from build123d import *

# Parameters (mm, degrees)
SKETCH_1_R             = 4
SKETCH_1_R_2           = 1.5
SKETCH_1_R_3           = 13
SM_BASE_FLANGE_1_DEPTH = 3


# Sheet-metal steps are written as plain solids
with BuildPart() as part:
    # Sketch 1 → 基体-法兰1 (new body)
    with BuildSketch(Plane(origin=(0, 0, 0), x_dir=(1, 0, 0), z_dir=(0, 1, 0))):
        with BuildLine():
            Line((23, 200), (23, 0))
            ThreePointArc((23, 0), (0, -23), (-23, 0))
            Line((-23, 0), (-23, 200))
            ThreePointArc((-23, 200), (0, 223), (23, 200))
        make_face()
        with Locations(Location((0, 0, 0), (0, 0, 270))):
            Circle(SKETCH_1_R, mode=Mode.SUBTRACT)
        with Locations(Location((-10, 35, 0), (0, 0, 270))):
            Circle(SKETCH_1_R_2, mode=Mode.SUBTRACT)
        with Locations(Location((10, 35, 0), (0, 0, 270))):
            Circle(SKETCH_1_R_2, mode=Mode.SUBTRACT)
        with Locations(Location((-10, 135, 0), (0, 0, 270))):
            Circle(SKETCH_1_R_2, mode=Mode.SUBTRACT)
        with Locations(Location((10, 135, 0), (0, 0, 270))):
            Circle(SKETCH_1_R_2, mode=Mode.SUBTRACT)
        with Locations(Location((0, 200, 0), (0, 0, 270))):
            Circle(SKETCH_1_R_3, mode=Mode.SUBTRACT)
        with Locations(Location((15, 0, 0), (0, 0, 270))):
            Circle(SKETCH_1_R_2, mode=Mode.SUBTRACT)
        with Locations(Location((-15, 0, 0), (0, 0, 270))):
            Circle(SKETCH_1_R_2, mode=Mode.SUBTRACT)
        with Locations(Location((0, 218, 0), (0, 0, 270))):
            Circle(SKETCH_1_R_2, mode=Mode.SUBTRACT)
        with Locations(Location((18, 200, 0), (0, 0, 270))):
            Circle(SKETCH_1_R_2, mode=Mode.SUBTRACT)
        with Locations(Location((0, 182, 0), (0, 0, 270))):
            Circle(SKETCH_1_R_2, mode=Mode.SUBTRACT)
        with Locations(Location((-18, 200, 0), (0, 0, 270))):
            Circle(SKETCH_1_R_2, mode=Mode.SUBTRACT)
        with BuildLine():
            Line((-8.5, 173), (-8.5, 163))
            ThreePointArc((-8.5, 163), (-10, 161.5), (-11.5, 163))
            Line((-11.5, 163), (-11.5, 173))
            ThreePointArc((-11.5, 173), (-10, 174.5), (-8.5, 173))
        make_face(mode=Mode.SUBTRACT)
        with BuildLine():
            Line((8.5, 163), (8.5, 173))
            ThreePointArc((8.5, 173), (10, 174.5), (11.5, 173))
            Line((11.5, 173), (11.5, 163))
            ThreePointArc((11.5, 163), (10, 161.5), (8.5, 163))
        make_face(mode=Mode.SUBTRACT)
    extrude(amount=-SM_BASE_FLANGE_1_DEPTH)


solid = part.part
Here's how the part is built. I have some questions about the finished solid (model axes, mm). Round coordinates to 2 decimals unless told otherwise and drop trailing zeros. Return JSON: item names as keys, results as strings. Group by question number.
1. If we mould it in two halves opening along X, with no side actions, what happens to faces 1 (the face through (-5, -1, -188)), 2 (the face through (0.506, -1.479, 22.994)), 3 (the face through (0, -3, -102)), 4 (the face through (-3.905, -1.479, -0.867))? For each: pulls with the +X half, pulls with the -X half, needs draft (parallel to the pull), parting line crosses it, or undercut.
2. Please list where these lines run through material, in increasing order: probe 1 along X at (y, z) = (-1.45, -200); probe 2 along X at (y, z) = (-1.65, -135); probe 3 along Z at (x, y) = (2.5, -2.15).
3. If we section it at A-A on y = -2.45: State how many separate pieces and enclosed holes the cut face has, then the cut area to 3 significant figures.
4. I'm going to push flat-ended pins straight in: pin 1 Ø4 at (x, z) = (15, 0) entering from -Y; pin 2 Ø23.5 at (x, z) = (0, -200) entering from -Y. Where does each tip first touch, or does it pass through?
Reply:
{
 "1": {"face 1": "undercut", "face 2": "parting line crosses it", "face 3": "needs draft", "face 4": "undercut"},
 "2": {"probe 1": "-23 to -19.5, -16.5 to -13, 13 to 16.5, 19.5 to 23", "probe 2": "-23 to -11.5, -8.5 to 8.5, 11.5 to 23", "probe 3": "-222.86 to -212.76, -187.24 to -3.12, 3.12 to 22.86"},
 "3": {"separate pieces": "1", "enclosed holes": "14", "area": "10,100 mm^2"},
 "4": {"pin 1": "y = -3", "pin 2": "through"}
}
